The listing builds one solid part. Answer for the finished solid, in the listing's coordinates (mm). A direction names the side the tool comes from. Give positions to 0.01 mm unless a question says otherwise; leave off trailing zeros. Loops run counter-clockwise (first coordinate to the right, second up) from the corner with the lowest first, then second, coordinate; pieces in that order, holes last. Notation, with made-up numbers: (-22.75, 23) - (-10.75, 23) arc R24 ccw to (-10.75, 55) - close; hole circle Ø5 at (61.5, -14). An arc over 180 degrees is marked (long way). One line per item, written item: value. Start each with the question number.
Autodesk Inventor part; units mm, degrees
ref_plane "YZ Plane" through (0, 0, 0) normal (1, 0, 0) x (0, 1, 0)
ref_plane "XZ Plane" through (0, 0, 0) normal (0, 1, 0) x (-1, 0, 0)
ref_plane "XY Plane" through (0, 0, 0) normal (0, 0, 1) x (1, 0, 0)
sketch "Sketch1" plane through (0, 0, 0) normal (0, 0, 1) x (1, 0, 0)
  line L0 (-28.575, -28.575) -> (28.575, -28.575)
  line L1 (28.575, -28.575) -> (28.575, 28.575)
  line L2 (28.575, 28.575) -> (-28.575, 28.575)
  line L3 (-28.575, 28.575) -> (-28.575, -28.575)
  line L4 (-28.575, -28.575) -> (28.575, 28.575) construction
  line L5 (28.575, -28.575) -> (-28.575, 28.575) construction
  point P0 (0, 0)
  dimension "d0" = 57.15
  dimension "d1" = 57.15
extrude "Extrusion1" add sketch "Sketch1" along normal blind 12.7
sketch "Sketch2" plane through (0, 0, 12.7) normal (0, 0, 1) x (1, 0, 0)
  line L0 (-21.15, -21.15) -> (21.15, -21.15)
  line L1 (21.15, -21.15) -> (21.15, 21.15)
  line L2 (21.15, 21.15) -> (-21.15, 21.15)
  line L3 (-21.15, 21.15) -> (-21.15, -21.15)
  line L4 (-21.15, -21.15) -> (21.15, 21.15) construction
  line L5 (21.15, -21.15) -> (-21.15, 21.15) construction
  point P0 (0, 0)
  dimension "d4" = 42.3
  dimension "d5" = 42.3
extrude "Extrusion2" cut sketch "Sketch2" against normal blind 6.35
sketch "Sketch3" plane through (0, 0, 0) normal (0, 0, -1) x (-1, 0, 0)
  line L0 (-15.5, -15.5) -> (15.5, -15.5) construction
  line L1 (15.5, -15.5) -> (15.5, 15.5) construction
  line L2 (15.5, 15.5) -> (-15.5, 15.5) construction
  line L3 (-15.5, 15.5) -> (-15.5, -15.5) construction
  line L4 (-15.5, -15.5) -> (15.5, 15.5) construction
  line L5 (15.5, -15.5) -> (-15.5, 15.5) construction
  point P0 (0, 0)
  dimension "d8" = 31
  dimension "d9" = 31
hole "Hole1" at (15.5, 15.5, 0) at (-15.5, 15.5, 0) at (-15.5, -15.5, 0) at (15.5, -15.5, 0) direction (0, 0, 1) diameter 3.2004 end through all
sketch "Sketch4" plane through (0, 0, 0) normal (0, 0, -1) x (-1, 0, 0)
  point P0 (0, 0)
  point P1 (0, 0)
sketch "Sketch5" plane through (0, 0, 6.35) normal (0, 0, 1) x (1, 0, 0)
  circle A0 centre (0, 0) radius 11
  dimension "d17" = 22
extrude "Extrusion3" cut sketch "Sketch5" against normal blind 2
hole "Hole2" at (0, 0, 0) direction (0, 0, 1) diameter 7 end through all
sketch "Sketch6" plane through (-28.575, -28.575, 0) normal (0, -1, 0) x (1, 0, 0)
  line L0 (57.15, 0) -> (57.15, 12.7)
  line L1 (0, 12.7) -> (57.15, 12.7)
  line L2 (0, 0) -> (0, 12.7)
  line L3 (28.575, 12.7) -> (28.575, 0) construction
  line L4 (0, 0) -> (57.15, 0)
  line L5 (10.16, 4.7625) -> (46.99, 4.7625) construction
  dimension "d27" = 12.7
  dimension "d28" = 10.16
  dimension "d29" = 10.16
  dimension "d45" = 7.9375
hole "Hole3" at (-18.415, -28.575, 4.7625) at (18.415, -28.575, 4.7625) direction (0, 1, 0) diameter 4.3434 depth 6.35 tip angle 118
sketch "Sketch7" plane through (0, 0, 12.7) normal (0, 0, 1) x (1, 0, 0)
  line L0 (-21.15, 21.15) -> (21.15, 21.15)
  line L1 (-28.575, -28.575) -> (28.575, -28.575)
  line L2 (28.575, 28.575) -> (-28.575, 28.575)
  line L3 (28.575, -28.575) -> (-28.575, 28.575) construction
  line L4 (28.575, 28.575) -> (-28.575, -28.575) construction
  line L5 (0, 28.575) -> (0, 21.15) construction
  line L6 (0, 24.8625) -> (24.8625, 24.8625) construction
  line L7 (-24.8625, -24.8625) -> (24.8625, -24.8625) construction
  line L8 (24.8625, -24.8625) -> (24.8625, 24.8625) construction
  line L9 (24.8625, 24.8625) -> (-24.8625, 24.8625) construction
  line L10 (-24.8625, 24.8625) -> (-24.8625, -24.8625) construction
  line L11 (-24.8625, -24.8625) -> (24.8625, 24.8625) construction
  line L12 (24.8625, -24.8625) -> (-24.8625, 24.8625) construction
  point P0 (0, 0)
hole "Hole4" at (-24.8625, 24.8625, 12.7) at (24.8625, 24.8625, 12.7) at (24.8625, -24.8625, 12.7) at (-24.8625, -24.8625, 12.7) direction (0, 0, -1) diameter 3.9624 depth 5.588 tip angle 118
equation "\"d29\" = d28"
properties part number "NEMA_17-front" material "Aluminum 6061"
1. A cutting plane is placed at D-D (z = 11.25). Give the number of separate pieces and of enclosed holes in the cut face, plus the area to 3 significant figures.
2. For faces 4 (the cylindrical face through (-14.08, 16.24, 3.22)), 5 (the cylindrical face through (-19.1, -25.4, 2.7)), 6 (the flat face through (-21.15, 0, 10)), determine the directions among +Z, -Z, +X, -X, +Y, -Y from which every point of the face is accessible in a straight line to the end or side of a thin tool.
3. Find the intervals of material crossed by L1, parallel to Y at x = -15.5, z = 3.25 (3 decimals); L2, parallel to Y at x = 10.5, z = 6.75 (3 decimals); L3, parallel to Y at x = 0, z = 2.75 (3 decimals), in increasing order. Write a range as [from, to].
4. A cutting plane is placed at A-A (x = 0). Determine the outline of the cut face in (y, z) (3 decimals), plus the area to 3 significant figures.
5. A cutting plane is placed at B-B (y = -15.5). Determine the outline of the cut face in (x, z) (3 decimals), plus the area to 3 significant figures.
6. Determine the mould class of faces 1 (the flat face through (0, -28.575, 6)), 2 (the flat face through (0, 28.575, 6)), 3 (the cylindrical face through (-22.93, -24.43, 9.87)) for opening direction Y: released by +Y, released by -Y, zero draft, split by the parting line, or undercut.
7. Flat-ended cylindrical pins translate along their axes: pin 1 (2 mm diameter, centred on x = -1.5, y = 16, fed in from +Z); pin 2 (4.5 mm diameter, centred on x = 24.86, y = 24.86, fed in from -Z); pin 3 (17.5 mm diameter, centred on x = -0.5, y = 1.5, fed in from +Z); pin 4 (3 mm diameter, centred on x = 15.5, y = 15.5, fed in from -Z). Find the tip coordinate at first contact, or state that the pin passes through.
Results below:
1. separate pieces: 1
1. enclosed holes: 5
1. area: 1,430 mm^2
2. face 4: +Z, -Z
2. face 5: -Y
2. face 6: +Z
3. L1: y = [-28.575, -17.1], [-13.9, 13.9], [17.1, 28.575]
3. L2: y = [-28.575, -21.15], [21.15, 28.575]
3. L3: y = [-28.575, -3.5], [3.5, 28.575]
4. outline: (-28.575, 0) - (-3.5, 0) - (-3.5, 4.35) - (-11, 4.35) - (-11, 6.35) - (-21.15, 6.35) - (-21.15, 12.7) - (-28.575, 12.7) - close; (3.5, 0) - (28.575, 0) - (28.575, 12.7) - (21.15, 12.7) - (21.15, 6.35) - (11, 6.35) - (11, 4.35) - (3.5, 4.35) - close
4. area: 383 mm^2
5. outline: (-28.575, 0) - (-17.1, 0) - (-17.1, 6.35) - (-21.15, 6.35) - (-21.15, 12.7) - (-28.575, 12.7) - close; (-13.9, 0) - (13.9, 0) - (13.9, 6.35) - (-13.9, 6.35) - close; (17.1, 0) - (28.575, 0) - (28.575, 12.7) - (21.15, 12.7) - (21.15, 6.35) - (17.1, 6.35) - close
5. area: 417 mm^2
6. face 1: released by -Y
6. face 2: released by +Y
6. face 3: undercut
7. pin 1: stops at z = 6.35
7. pin 2: stops at z = 0
7. pin 3: stops at z = 4.35
7. pin 4: passes through
